```python
from build123d import *

# Parameters (mm, degrees)
F1_DEPTH    = 76.2
F2_SIZE     = 5.08
F3_SIZE     = 5.08
F4_SIZE     = 5.08
F5_T1_DEPTH = 92.1682991577
F5_T3_DEPTH = 133.3862799398
F5_T5_DEPTH = 77.5062799398


# Not quite as in the source:
# - a fillet or chamfer that OpenCascade refuses, or shapes differently, is made with other operations: its cross-section is extruded or revolved along the edge and cut away or added


with BuildPart() as f1:
    # F0 (on Front) → F1 (new body)
    with BuildSketch(Plane.XZ):
        Polygon((-5.919593852, -19.1378965259), (13.130406148, -19.1378965259), (13.130406148, 107.8621034741), (-5.919593852, 107.8621034741), (-5.919593852, 82.4621034741), (3.605406148, 82.4621034741), (3.605406148, 63.4121034741), (-5.919593852, 63.4121034741), align=None)
    extrude(amount=F1_DEPTH)

    # F2
    f2_edges = [f1.edges().sort_by_distance(p)[0] for p in [
        (-5.919594, 0, 95.162103),
        (13.130406, 0, 44.362103),
        (3.605406, 0, -19.137897),
        (-5.919594, 0, 22.137103),
        (-5.919594, -38.1, -19.137897),
        (-5.919594, -76.2, 22.137103),
        (13.130406, -38.1, -19.137897),
        (3.605406, -76.2, -19.137897),
        (13.130406, -76.2, 44.362103),
        (3.605406, -76.2, 107.862103),
        (-5.919594, -38.1, 107.862103),
    ]]
    chamfer(f2_edges, length=F2_SIZE)

    # F3
    f3_edges = [f1.edges().sort_by_distance(p)[0] for p in [
        (-5.919594, -76.2, 92.622103),
    ]]
    chamfer(f3_edges, length=F3_SIZE)

    # F4
    f4_edges = [f1.edges().sort_by_distance(p)[0] for p in [
        (3.605406, 0, 107.862103),
    ]]
    chamfer(f4_edges, length=F4_SIZE)

    # F5: chamfer of 5.08 on 4 edges, made by hand

    # F5_s2 → F5_t1 (cut)
    with BuildSketch(Plane.XZ.offset(-7.9841495789)):
        Polygon((8.050406148, 107.8621034741), (13.130406148, 102.7821034741), (13.130406148, 107.8621034741), align=None)
    extrude(amount=F5_T1_DEPTH, mode=Mode.SUBTRACT)

    # F5_s4 → F5_t3 (cut)
    with BuildSketch(Plane.XY.offset(-19.7910364957)):
        Polygon((13.130406148, -69.0157951031), (11.6425085964, -72.6078975516), (13.130406148, -71.12), align=None)
        Polygon((11.6425085964, -3.5921024484), (13.130406148, -7.1842048969), (13.130406148, -5.08), align=None)
    extrude(amount=F5_T3_DEPTH, mode=Mode.SUBTRACT)

    # F5_s6 → F5_t5 (cut)
    with BuildSketch(Plane.XZ.offset(-0.6531399699)):
        Polygon((13.130406148, -11.953691629), (11.6425085964, -15.5457940774), (13.130406148, -14.0578965259), align=None)
    extrude(amount=F5_T5_DEPTH, mode=Mode.SUBTRACT)


solid = f1.part
```
Source: CAD feature listing. Evaluate the final solid. Frame: model axes, mm. A direction names the side the tool comes from. Give positions to 0.01 mm unless a question says otherwise; leave off trailing zeros. Write each loop counter-clockwise with the first axis right and the second up, starting at its lowest first coordinate (ties: lowest second). Pieces come first, ordered by that corner, then holes. Notation, with made-up numbers: (8.25, 79) - (29.25, 79) arc R15 cw to (29.25, 90) - close; hole circle Ø9 at (65.5, -20.5). An arc over 180 degrees is marked (long way). One line per item, written item: value. Start each with the question number.
Q1. Section query C-C, the plane y = -11.5. Return the cut outline in (x, z).
Q2. Section query B-B, the plane z = 71.5. Return the cut outline in (x, y).
Q3. Section query A-A, the plane x = 2. Return the cut outline in (y, z), then the cut area to 3 significant figures.
Q4. Section query D-D, the plane z = 2. Return the cut outline in (x, y), then the cut area to 3 significant figures.
Q5. Material intervals for probe 1 along Z at (x, y) = (0, -38); probe 2 along Z at (x, y) = (-1.25, -57); probe 3 along X at (y, z) = (-21.5, 80), sorted ascending. Write a range as from..to.
Q6. First-contact query: pin 1 Ø5 at (x, y) = (-1, -52.5) entering from +Z; pin 2 Ø9.5 at (y, z) = (-31, 70.5) entering from -X. Flat tips, straight axial feed; report the tip coordinate or a pass-through.
Q7. Set-up query: faces 1 (the face through (-1, -38, 63.412)), 2 (the face through (-2.8, -3.5, -15.6)). Return all of +Z, -Z, +X, -X, +Y, -Y with unobstructed straight access to the full face (end or side cutting, diameter ignored); none if empty.
Answer:
1. outline: (-5.92, -14.06) - (-0.84, -19.14) - (8.05, -19.14) - (11.64, -15.55) - (13.13, -11.95) - (13.13, 102.78) - (8.05, 107.86) - (-0.84, 107.86) - (-5.92, 102.78) - (-5.92, 82.46) - (3.61, 82.46) - (3.61, 63.41) - (-5.92, 63.41) - close
2. outline: (3.61, -76.2) - (8.05, -76.2) - (11.64, -72.61) - (13.13, -69.02) - (13.13, -7.18) - (11.64, -3.59) - (8.05, 0) - (3.61, 0) - close
3. outline: (-76.2, -14.06) - (-71.12, -19.14) - (-5.08, -19.14) - (0, -14.06) - (0, 63.41) - (-76.2, 63.41) - close; (-76.2, 82.46) - (0, 82.46) - (0, 102.78) - (-5.08, 107.86) - (-71.12, 107.86) - (-76.2, 102.78) - close
3. area: 8,170 mm2
4. outline: (-5.92, -71.12) - (-0.84, -76.2) - (8.05, -76.2) - (11.64, -72.61) - (13.13, -69.02) - (13.13, -7.18) - (11.64, -3.59) - (8.05, 0) - (-0.84, 0) - (-5.92, -5.08) - close
4. area: 1,400 mm2
5. probe 1: z = -19.14..63.41, 82.46..107.86
5. probe 2: z = -18.73..63.41, 82.46..107.45
5. probe 3: x = 3.61..13.13
6. pin 1: stops at z = 107.86
6. pin 2: stops at x = 3.61
7. face 1: -X, +Y, -Y
7. face 2: -Z, -X, +Y
